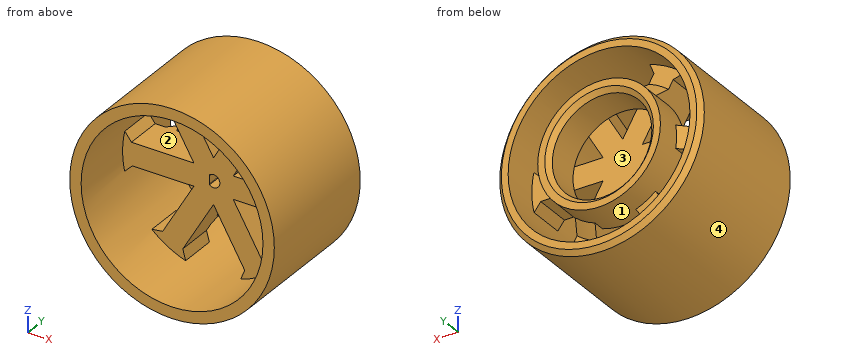
```python
from build123d import *

# Parameters (mm, degrees)
SKETCH1_R               = 22.5
SKETCH1_R_2             = 20
BOSS_EXTRUDE1_DEPTH     = 30
BOSS_EXTRUDE2_DEPTH     = 4
CHAMFER1_SIZE           = 2
CHAMFER1_SIZE_2         = 1.79025908
CUT_EXTRUDE1_DEPTH      = 39.684622268
CUT_EXTRUDE1_DEPTH_BACK = 39.684622268
BOSS_EXTRUDE3_START     = -1.5
BOSS_EXTRUDE3_DEPTH     = 1.5
SKETCH6_R               = 13.5
SKETCH6_R_2             = 10.95
BOSS_EXTRUDE4_DEPTH     = 8
CHAMFER2_SIZE           = 1
CHAMFER3_SIZE           = 1
CHAMFER4_SIZE           = 2.5


with BuildPart() as part:
    # Sketch1 → Boss-Extrude1 (new body)
    with BuildSketch(Plane(origin=(0, 0, 0), x_dir=(1, 0, 0), z_dir=(0, 1, 0))):
        with Locations(Location((0, 0, 0), (0, 0, 270))):
            Circle(SKETCH1_R)
        with Locations(Location((0, 0, 0), (0, 0, 270))):
            Circle(SKETCH1_R_2, mode=Mode.SUBTRACT)
    extrude(amount=BOSS_EXTRUDE1_DEPTH)

    # Sketch2 → Boss-Extrude2 (add, symmetric)
    with BuildSketch(Plane(origin=(0, 18, 0), x_dir=(1, 0, 0), z_dir=(0, 1, 0))):
        with BuildLine():
            Line((-12.086630926, 15.934658856), (-4.330127019, 2.5))
            Line((-4.330127019, 2.5), (-19.843134833, 2.5))
            ThreePointArc((-19.843134833, 2.5), (-20, 0), (-19.843134833, -2.5))
            Line((-19.843134833, -2.5), (-4.330127019, -2.5))
            Line((-4.330127019, -2.5), (-12.086630926, -15.934658856))
            ThreePointArc((-12.086630926, -15.934658856), (-10, -17.320508076), (-7.756503907, -18.434658856))
            Line((-7.756503907, -18.434658856), (0, -5))
            Line((0, -5), (7.756503907, -18.434658856))
            ThreePointArc((7.756503907, -18.434658856), (10, -17.320508076), (12.086630926, -15.934658856))
            Line((12.086630926, -15.934658856), (4.330127019, -2.5))
            Line((4.330127019, -2.5), (19.843134833, -2.5))
            ThreePointArc((19.843134833, -2.5), (19.960745185, -1.252458251), (20, 0))
            ThreePointArc((20, 0), (19.960745185, 1.252458251), (19.843134833, 2.5))
            Line((19.843134833, 2.5), (4.330127019, 2.5))
            Line((4.330127019, 2.5), (12.086630926, 15.934658856))
            ThreePointArc((12.086630926, 15.934658856), (10, 17.320508076), (7.756503907, 18.434658856))
            Line((7.756503907, 18.434658856), (0, 5))
            Line((0, 5), (-7.756503907, 18.434658856))
            ThreePointArc((-7.756503907, 18.434658856), (-10, 17.320508076), (-12.086630926, 15.934658856))
        make_face()
    extrude(amount=BOSS_EXTRUDE2_DEPTH, both=True)

    # Chamfer1
    # the kernel refuses this chamfer: 2, 1.79025908 mm, written as the material it adds along each edge
    with BuildSketch(Plane(origin=(7.756503907, 22, 18.434658856), x_dir=(-0.9376749432180777, 0, 0.34751359809505994), z_dir=(0, -1, 0)), Plane(origin=(19.843134833, 22, 2.5), x_dir=(-0.16788186749818226, 0, 0.9858071203665161), z_dir=(0, -1, 0)), Plane(origin=(12.086630926, 22, -15.934658856), x_dir=(0.7697930757198956, 0, 0.6382935222714571), z_dir=(0, -1, 0)), Plane(origin=(-7.756503907, 22, -18.434658856), x_dir=(0.9376749432180783, 0, -0.34751359809505833), z_dir=(0, -1, 0)), Plane(origin=(-19.843134833, 22, -2.5), x_dir=(0.1678818674981782, 0, -0.9858071203665167), z_dir=(0, -1, 0)), Plane(origin=(-12.086630926, 22, 15.934658856), x_dir=(-0.7697930757198955, 0, -0.6382935222714572), z_dir=(0, -1, 0))) as chamfer1_piece_1:
        with BuildLine():
            Line((1.733569464, 0), (CHAMFER1_SIZE * 0.167881867498, CHAMFER1_SIZE * 0.985807120367))
            Line((CHAMFER1_SIZE * 0.167881867498, CHAMFER1_SIZE * 0.985807120367), (0, 0))
            ThreePointArc((0, 0), (0.889903139, -0.018778361), (1.733569464, 0))
        make_face()
    extrude(amount=8)
    with BuildSketch(Plane(origin=(12.086630926, 14, 15.934658856), x_dir=(0.7669529363679002, 0, -0.6417033531131466), z_dir=(0, 1, 0)), Plane(origin=(19.843134833, 14, -2.5), x_dir=(-0.17225493730569186, 0, -0.9850524029582447), z_dir=(0, 1, 0)), Plane(origin=(7.756503907, 14, -18.434658856), x_dir=(-0.9392078736735914, 0, -0.3433490498450975), z_dir=(0, 1, 0)), Plane(origin=(-12.086630926, 14, -15.934658856), x_dir=(-0.766952936367899, 0, 0.641703353113148), z_dir=(0, 1, 0)), Plane(origin=(-19.843134833, 14, 2.5), x_dir=(0.17225493730568892, 0, 0.9850524029582453), z_dir=(0, 1, 0)), Plane(origin=(-7.756503907, 14, 18.434658856), x_dir=(0.9392078736735913, 0, 0.3433490498450977), z_dir=(0, 1, 0))) as chamfer1_piece_2:
        with BuildLine():
            Line((1.910893878, 0), (CHAMFER1_SIZE_2 * 0.172254937261, CHAMFER1_SIZE_2 * 0.985052402702))
            Line((CHAMFER1_SIZE_2 * 0.172254937261, CHAMFER1_SIZE_2 * 0.985052402702), (0, 0))
            ThreePointArc((0, 0), (0.982338586, -0.022816928), (1.910893878, 0))
        make_face()
    extrude(amount=8)

    # Sketch4 → Cut-Extrude1 (cut, two sides: drawn at the far end of the back side and taken through both)
    with BuildSketch(Plane(origin=(0, 22, 0), x_dir=(1, 0, 0), z_dir=(0, 1, 0)).offset(-CUT_EXTRUDE1_DEPTH_BACK)):
        with BuildLine():
            Line((-0.896831774, 1.07503152), (-0.897545019, 0.833314429))
            Line((-0.897545019, 0.833314429), (-0.902447145, -0.828003111))
            Line((-0.902447145, -0.828003111), (-0.90316039, -1.069720202))
            ThreePointArc((-0.90316039, -1.069720202), (1.399993905, -0.004131026), (-0.896831774, 1.07503152))
        make_face()
    extrude(amount=CUT_EXTRUDE1_DEPTH + CUT_EXTRUDE1_DEPTH_BACK, mode=Mode.SUBTRACT)

    # Sketch5 → Boss-Extrude3 (add)
    with BuildSketch(Plane(origin=(0, 22, 0), x_dir=(1, 0, 0), z_dir=(0, 1, 0)).offset(BOSS_EXTRUDE3_START)):
        with BuildLine():
            Line((-0.896831774, 1.07503152), (-0.90316039, -1.069720202))
            ThreePointArc((-0.90316039, -1.069720202), (1.399993905, -0.004131026), (-0.896831774, 1.07503152))
        make_face()
    extrude(amount=BOSS_EXTRUDE3_DEPTH)

    # Sketch6 → Boss-Extrude4 (add)
    with BuildSketch(Plane(origin=(0, 22, 0), x_dir=(1, 0, 0), z_dir=(0, 1, 0))):
        with Locations(Location((0, 0, 0), (0, 0, 109.328070714))):
            Circle(SKETCH6_R)
        with Locations(Location((0, 0, 0), (0, 0, 106.802375663))):
            Circle(SKETCH6_R_2, mode=Mode.SUBTRACT)
    extrude(amount=BOSS_EXTRUDE4_DEPTH)

    # Chamfer2
    chamfer2_edges = [part.edges().sort_by_distance(p)[0] for p in [
        (0, 30, -22.5),
    ]]
    chamfer(chamfer2_edges, length=CHAMFER2_SIZE)

    # Chamfer3
    chamfer3_edges = [part.edges().sort_by_distance(p)[0] for p in [
        (3.165332817, 30, 10.482517262),
    ]]
    chamfer(chamfer3_edges, length=CHAMFER3_SIZE)

    # Chamfer4
    # the kernel refuses this chamfer: 2.5 mm, written as the material it adds along each edge
    with BuildSketch(Plane(origin=(0, 22, 0), x_dir=(0.7884516512749685, 0, 0.6150967351577924), z_dir=(-0.6150967351577924, 0, 0.7884516512749685))) as chamfer4_piece_1_section:
        Polygon((13.5, CHAMFER4_SIZE), (13.5 + CHAMFER4_SIZE, 0), (13.5, 0), align=None)
    chamfer4_piece_1 = revolve(axis=Axis((0, 22, 0), (0, 1, 0)), revolution_arc=75.917899148, mode=Mode.PRIVATE)
    chamfer4_piece_1 = split(chamfer4_piece_1, bisect_by=Plane(origin=(0, 22, 2.5), z_dir=(0, 0, -1)), keep=Keep.TOP, mode=Mode.PRIVATE)
    chamfer4_piece_1 = split(chamfer4_piece_1, bisect_by=Plane(origin=(0, 22, -2.5), z_dir=(0, 0, 1)), keep=Keep.TOP, mode=Mode.PRIVATE)
    add(chamfer4_piece_1)
    with BuildSketch(Plane(origin=(0, 22, 0), x_dir=(0.9269152240690147, 0, -0.3752707920809829), z_dir=(0.3752707920809829, 0, 0.9269152240690147))) as chamfer4_piece_2_section:
        Polygon((13.5, CHAMFER4_SIZE), (13.5 + CHAMFER4_SIZE, 0), (13.5, 0), align=None)
    chamfer4_piece_2 = revolve(axis=Axis((0, 22, 0), (0, 1, 0)), revolution_arc=75.917899148, mode=Mode.PRIVATE)
    chamfer4_piece_2 = split(chamfer4_piece_2, bisect_by=Plane(origin=(2.165063509, 22, 1.25), z_dir=(-0.8660254037844385, 0, -0.5000000000000003)), keep=Keep.TOP, mode=Mode.PRIVATE)
    chamfer4_piece_2 = split(chamfer4_piece_2, bisect_by=Plane(origin=(-2.165063509, 22, -1.25), z_dir=(0.8660254037844383, 0, 0.5000000000000009)), keep=Keep.TOP, mode=Mode.PRIVATE)
    add(chamfer4_piece_2)
    with BuildSketch(Plane(origin=(0, 22, 0), x_dir=(0.138463572798161, 0, -0.9903675272382311), z_dir=(0.9903675272382311, 0, 0.138463572798161))) as chamfer4_piece_3_section:
        Polygon((13.5, CHAMFER4_SIZE), (13.5 + CHAMFER4_SIZE, 0), (13.5, 0), align=None)
    chamfer4_piece_3 = revolve(axis=Axis((0, 22, 0), (0, 1, 0)), revolution_arc=75.917899148, mode=Mode.PRIVATE)
    chamfer4_piece_3 = split(chamfer4_piece_3, bisect_by=Plane(origin=(-2.165063509, 22, 1.25), z_dir=(0.8660254037844393, 0, -0.49999999999999906)), keep=Keep.TOP, mode=Mode.PRIVATE)
    chamfer4_piece_3 = split(chamfer4_piece_3, bisect_by=Plane(origin=(2.165063509, 22, -1.25), z_dir=(-0.8660254037844392, 0, 0.49999999999999917)), keep=Keep.TOP, mode=Mode.PRIVATE)
    add(chamfer4_piece_3)
    with BuildSketch(Plane(origin=(0, 22, 0), x_dir=(-0.788451651274934, 0, -0.6150967351578366), z_dir=(0.6150967351578366, 0, -0.788451651274934))) as chamfer4_piece_4_section:
        Polygon((13.5, CHAMFER4_SIZE), (13.5 + CHAMFER4_SIZE, 0), (13.5, 0), align=None)
    chamfer4_piece_4 = revolve(axis=Axis((0, 22, 0), (0, 1, 0)), revolution_arc=75.917899148, mode=Mode.PRIVATE)
    chamfer4_piece_4 = split(chamfer4_piece_4, bisect_by=Plane(origin=(0, 22, -2.5), z_dir=(0, 0, 1)), keep=Keep.TOP, mode=Mode.PRIVATE)
    chamfer4_piece_4 = split(chamfer4_piece_4, bisect_by=Plane(origin=(0, 22, 2.5), z_dir=(0, 0, -1)), keep=Keep.TOP, mode=Mode.PRIVATE)
    add(chamfer4_piece_4)
    with BuildSketch(Plane(origin=(0, 22, 0), x_dir=(-0.9269152240690146, 0, 0.375270792080983), z_dir=(-0.375270792080983, 0, -0.9269152240690146))) as chamfer4_piece_5_section:
        Polygon((13.5, CHAMFER4_SIZE), (13.5 + CHAMFER4_SIZE, 0), (13.5, 0), align=None)
    chamfer4_piece_5 = revolve(axis=Axis((0, 22, 0), (0, 1, 0)), revolution_arc=75.917899148, mode=Mode.PRIVATE)
    chamfer4_piece_5 = split(chamfer4_piece_5, bisect_by=Plane(origin=(-2.165063509, 22, -1.25), z_dir=(0.8660254037844384, 0, 0.5000000000000006)), keep=Keep.TOP, mode=Mode.PRIVATE)
    chamfer4_piece_5 = split(chamfer4_piece_5, bisect_by=Plane(origin=(2.165063509, 22, 1.25), z_dir=(-0.8660254037844386, 0, -0.5000000000000003)), keep=Keep.TOP, mode=Mode.PRIVATE)
    add(chamfer4_piece_5)
    with BuildSketch(Plane(origin=(0, 22, 0), x_dir=(-0.13846357279405325, 0, 0.9903675272388054), z_dir=(-0.9903675272388054, 0, -0.13846357279405325))) as chamfer4_piece_6_section:
        Polygon((13.5, CHAMFER4_SIZE), (13.5 + CHAMFER4_SIZE, 0), (13.5, 0), align=None)
    chamfer4_piece_6 = revolve(axis=Axis((0, 22, 0), (0, 1, 0)), revolution_arc=75.917899148, mode=Mode.PRIVATE)
    chamfer4_piece_6 = split(chamfer4_piece_6, bisect_by=Plane(origin=(-2.165063509, 22, 1.25), z_dir=(0.8660254037844392, 0, -0.4999999999999992)), keep=Keep.TOP, mode=Mode.PRIVATE)
    chamfer4_piece_6 = split(chamfer4_piece_6, bisect_by=Plane(origin=(2.165063509, 22, -1.25), z_dir=(-0.866025403784439, 0, 0.4999999999999993)), keep=Keep.TOP, mode=Mode.PRIVATE)
    add(chamfer4_piece_6)


solid = part.part
```
Read the model definition and answer for the solid it produces. Units are mm, in the model's axes. Face numbers are marked on the shaded views. A direction names the side the tool comes from. Coordinates: 2 decimals unless noted, no trailing zeros. Order: outer loops, then holes, each group sorted by start corner. A loop starts at its lowest first (then second) coordinate and runs counter-clockwise, first axis right, second up. Notation, with made-up numbers: (42.25, -3) - (50.25, -3) arc R31 cw to (50.25, 34) - close; hole circle Ø10 at (-30, -6). An arc over 180 degrees is marked (long way). Answer as a JSON object with one key per item and string values. Group by question number.
Item 1: A tool of negligible diameter and unlimited length cuts with its end or side. For the marked faces 1 and 2, from which of +Z, -Z, +X, -X, +Y, -Y can it reach the whole face along a straight path? Write none if from no direction.
Item 2: Flat-ended cylindrical pins translate along their axes: P1, Ø4.5, axis at x = 11.5, z = 6.5, coming from the -Y side; P2, Ø3, axis at x = -14, y = 20.5, coming from the +Z side; P3, Ø1.3, axis at x = -17.5, z = 0.5, coming from the +Y side. Find the tip coordinate at first contact, or state that the pin passes through.
Item 3: Section A-A (y = 21.25) is taken. State how many separate pieces and enclosed holes the cut face has, plus the area to 3 significant figures.
Item 4: Section D-D (y = 11) is taken. Give the vertices of the cut face in (x, z), plus the area to 3 significant figures.
Item 5: Consider probe 1 along X at (y, z) = (26.5, 0); probe 2 along X at (y, z) = (21.5, -3.5); probe 3 along X at (y, z) = (18, -4). Determine where each line is inside the solid, lowest interval first. Write a range as from..to.
Item 6: The mould has two halves that part along X. Classify the marked faces 3 and 4: +X half, -X half, draft (parallel to the pull), parting line (faces both ways), or undercut.
Item 7: Section B-B (y = 25.25) is taken. Give the vertices of the cut face in (x, z), plus the area to 3 significant figures.
Results are:
{
 "1": {"face 1": "+Y", "face 2": "-Y"},
 "2": {"P1": "stops at y = 22", "P2": "stops at z = 18.71", "P3": "stops at y = 22"},
 "3": {"separate pieces": "1", "enclosed holes": "6", "area": "888 mm^2"},
 "4": {"outline": "circle Ø45 at (0, 0); hole circle Ø40 at (0, 0)", "area": "334 mm^2"},
 "5": {"probe 1": "x = -22.5..-20, -13.5..-10.95, 10.95..13.5, 20..22.5", "probe 2": "x = -22.23..-18.84, -4.91..4.91, 18.83..22.23", "probe 3": "x = -22.14..-19.34, -5.2..5.2, 19.22..22.14"},
 "6": {"face 3": "undercut", "face 4": "parting line"},
 "7": {"outline": "circle Ø45 at (0, 0); circle Ø27 at (0, 0); hole circle Ø40 at (0, 0); hole circle Ø21.9 at (0, 0)", "area": "530 mm^2"}
}
